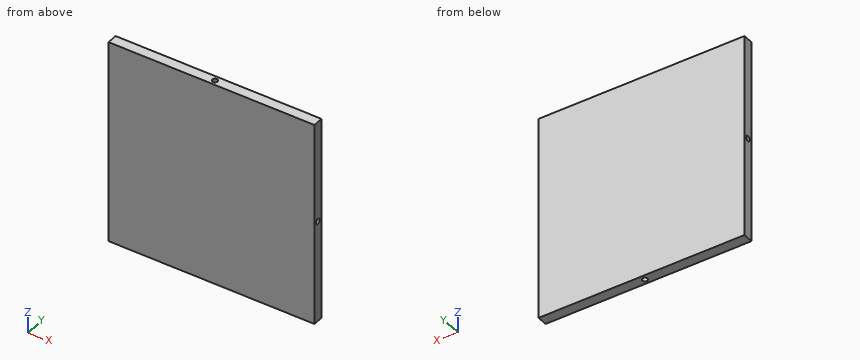
```python
from build123d import *

# Parameters (mm, degrees)
SKETCH_1_W          = 120
SKETCH_1_H          = 120
EXTRUDE_1_DEPTH     = 6
SKETCH_2_R          = 1.5
CUT_EXTRUDE_1_DEPTH = 16
SKETCH_3_R          = 1.5
CUT_EXTRUDE_4_DEPTH = 16
SKETCH_4_R          = 1.5
CUT_EXTRUDE_5_DEPTH = 16
SKETCH_5_R          = 1.5
CUT_EXTRUDE_6_DEPTH = 16


with BuildPart() as part:
    # 草图1 → 凸台-拉伸1 (new body)
    with BuildSketch(Plane(origin=(0, 0, 0), x_dir=(1, 0, 0), z_dir=(0, 1, 0))):
        Rectangle(SKETCH_1_W, SKETCH_1_H)
    extrude(amount=EXTRUDE_1_DEPTH)

    # 草图2 → 切除-拉伸1 (cut)
    with BuildSketch(Plane(origin=(60, 0, 0), x_dir=(0, 0, -1), z_dir=(1, 0, 0))):
        with Locations((0, 3)):
            Circle(SKETCH_2_R)
    extrude(amount=-CUT_EXTRUDE_1_DEPTH, mode=Mode.SUBTRACT)

    # 草图3 → 切除-拉伸4 (cut)
    with BuildSketch(Plane(origin=(0, 0, -60), x_dir=(-1, 0, 0), z_dir=(0, 0, -1))):
        with Locations((0, 3)):
            Circle(SKETCH_3_R)
    extrude(amount=-CUT_EXTRUDE_4_DEPTH, mode=Mode.SUBTRACT)

    # 草图4 → 切除-拉伸5 (cut)
    with BuildSketch(Plane.ZY.offset(60)):
        with Locations((0, 3)):
            Circle(SKETCH_4_R)
    extrude(amount=-CUT_EXTRUDE_5_DEPTH, mode=Mode.SUBTRACT)

    # 草图5 → 切除-拉伸6 (cut)
    with BuildSketch(Plane.XY.offset(60)):
        with Locations((0, 3)):
            Circle(SKETCH_5_R)
    extrude(amount=-CUT_EXTRUDE_6_DEPTH, mode=Mode.SUBTRACT)


solid = part.part
```
Work out the finished part from the listing and answer in its coordinate system (mm). Give positions to 0.01 mm unless a question says otherwise; leave off trailing zeros. Write each loop counter-clockwise with the first axis right and the second up, starting at its lowest first coordinate (ties: lowest second). Pieces come first, ordered by that corner, then holes. Notation, with made-up numbers: (-8, 10) -> (3, 10) arc R26 ccw to (3, 47) -> close; hole circle Ø4 at (42.25, 19.25). An arc over 180 degrees is marked (long way). Write each question's results on one line, items separated by ' | '.
1. Each of these flat-tipped pins is pushed along its axis until it touches: pin 1 Ø2.5 at (y, z) = (3, 0) entering from -X; pin 2 Ø1.8 at (x, y) = (0, 3) entering from -Z; pin 3 Ø2.5 at (y, z) = (3, 0) entering from +X. Where does it stop, or does it pass through?
Data:
pin 1: x = -44 | pin 2: z = -44 | pin 3: x = 44
2. Find section A-A on z = 0. Determine the outline of the cut face in (x, y).
Data:
outline: (-60, 0) -> (60, 0) -> (60, 1.5) -> (44, 1.5) -> (44, 4.5) -> (60, 4.5) -> (60, 6) -> (-60, 6) -> (-60, 4.5) -> (-44, 4.5) -> (-44, 1.5) -> (-60, 1.5) -> close
3. Straight lines are drawn through the part: L1, parallel to X at y = 2.9, z = -51; L2, parallel to Y at x = -56, z = 0. For each, find the intervals that lie inside material, in ascending order.
Data:
L1: -60 to -1.5, 1.5 to 60 | L2: 0 to 1.5, 4.5 to 6
4. Find section B-B on x = 0. Determine the outline of the cut face in (y, z), and give its area (3 significant figures).
Data:
outline: (0, -60) -> (1.5, -60) -> (1.5, -44) -> (4.5, -44) -> (4.5, -60) -> (6, -60) -> (6, 60) -> (4.5, 60) -> (4.5, 44) -> (1.5, 44) -> (1.5, 60) -> (0, 60) -> close | area: 624 mm^2
